```python
from build123d import *

# Parameters (mm, degrees)
BOSS_EXTRUDE1_DEPTH   = 1.6
F_4_CLEARANCE_HOLE1_D = 2.9464


with BuildPart() as part:
    # Sketch1 → Boss-Extrude1 (new body)
    with BuildSketch(Plane(origin=(0, 0, 0), x_dir=(1, 0, 0), z_dir=(0, 1, 0))):
        with BuildLine():
            Line((-37.5, -32.3215), (37.5, -32.3215))
            Line((37.5, -32.3215), (39.905002751, -56.11749224))
            Line((39.905002751, -56.11749224), (28.646672501, -62.61749224))
            ThreePointArc((28.646672501, -62.61749224), (0, -52.3215), (-28.646672501, -62.61749224))
            Line((-28.646672501, -62.61749224), (-39.905002751, -56.11749224))
            Line((-39.905002751, -56.11749224), (-37.5, -32.3215))
        make_face()
    extrude(amount=BOSS_EXTRUDE1_DEPTH)

    # #4 Clearance Hole1 (through all)
    with Locations(Plane(origin=(0, 1.6, 0), x_dir=(1, 0, 0), z_dir=(0, 1, 0))):
        with Locations((22.225, -38.494829198), (26.9875, -46.743721169), (31.75, -54.99261314)):
            f_4_clearance_hole1 = Hole(F_4_CLEARANCE_HOLE1_D / 2)

    # Mirror1: #4 Clearance Hole1 across plane
    add(f_4_clearance_hole1.mirror(Plane(origin=(0, 0, 0), x_dir=(0, 0, 1), z_dir=(1, 0, 0))), mode=Mode.SUBTRACT)


solid = part.part
```
Input: part model. Units: mm. Frame: model coordinates. Coordinates: 2 decimals unless noted, no trailing zeros. Loops run counter-clockwise (first coordinate to the right, second up) from the corner with the lowest first, then second, coordinate; pieces in that order, holes last.
Q1. Mould query, pull axis Z, two halves, no side actions, for faces 1 (the flat face through (1, 1.6, 44)), 2 (the cylindrical face through (32.84, 0.79, 54)), 3 (the flat face through (34.355, 0.789, 59.322)). Classes: +Z half, -Z half, draft (parallel to the pull), parting line (faces both ways), or undercut.
Results are:
face 1: draft
face 2: undercut
face 3: +Z half
Q2. Contact query for a flat-ended pin moving along its axis: pin 1 (8 mm diameter, centred on x = 20, z = 50, fed in from -Y). Output: stop coordinate, or through.
Results are:
pin 1: stops at y = 0
Q3. Section B-B, the plane y = 0.5. Give the number of separate pieces and of enclosed holes in the cut face, and give its area (3 significant figures).
Results are:
separate pieces: 1
enclosed holes: 6
area: 1,840 mm2
Q4. Section C-C, the plane x = -17.5. Return the cut outline in (y, z).
Results are:
outline: (0, 32.32) - (1.6, 32.32) - (1.6, 55.86) - (0, 55.86) - close
Q5. Line query: line 1 along X through (y, z) = (0.1, 48); line 2 along X through (y, z) = (0.85, 46); line 3 along X through (y, z) = (1.35, 55.5). Output: solid intervals per line, ascending.
Results are:
line 1: x = -39.08 to -27.76, -26.22 to 26.22, 27.76 to 39.08
line 2: x = -38.88 to -28.26, -25.72 to 25.72, 28.26 to 38.88
line 3: x = -39.84 to -33.13, -30.37 to -16.61, 16.61 to 30.37, 33.13 to 39.84
Q6. Section A-A, the plane x = 31.75. Return the cut outline in (y, z).
Results are:
outline: (0, 32.32) - (1.6, 32.32) - (1.6, 53.52) - (0, 53.52) - close; (0, 56.47) - (1.6, 56.47) - (1.6, 60.83) - (0, 60.83) - close
